For this review, take the finished solid that the model builds, in its own axes (mm). Round coordinates to 2 decimals unless told otherwise and drop trailing zeros. Loops run counter-clockwise (first coordinate to the right, second up) from the corner with the lowest first, then second, coordinate; pieces in that order, holes last. Notation, with made-up numbers: M -33,-22 L 1,-22 A20 ccw 1,6 Z; hole C -30,20.5 d9. An arc over 180 degrees is marked long. One line per question, with ' | ' between items. Start each with the question number.
1) We need section D-D (z = 15.5). Give the boundary of the cut face in (x, y), and give its area (3 significant figures).
2) For probe 1 along Z at (x, y) = (37.5, -1.25); probe 2 along X at (y, z) = (-0.25, 65); probe 3 along X at (y, z) = (-4, 45.5), list the stretches that pass through material, from the lowest coordinate up. Write a range as from..to.
3) For pin 1 Ø5 at (x, y) = (11, 2) entering from +Z; pin 2 Ø1 at (x, z) = (30, 11.5) entering from +Y; pin 3 Ø8 at (y, z) = (-3.5, 21.5) entering from +X, all flat-tipped, find the tip position at first contact; note any pin that passes through.
4) We need section B-B (y = 0). Give the boundary of the cut face in (x, z).
5) We need section A-A (x = 30). Give the boundary of the cut face in (y, z).
6) Mouldability with a two-part tool opening along X and no side actions: class faces 1 (the face through (0.57, 6.9, -0.08)), 2 (the face through (59.43, 0.08, -6.9)), 3 (the face through (25, 0, 40)), 4 (the face through (23, 0, 7.5)) as pulls with the +X half, pulls with the -X half, needs draft (parallel to the pull), parting line crosses it, or undercut.
7) We need section C-C (x = 48). Give the boundary of the cut face in (y, z).
```python
from build123d import *

# Parameters (mm, degrees)
SKETCH1_W           = 15
SKETCH1_H           = 15
BOSS_EXTRUDE1_DEPTH = 60
SKETCH3_R           = 5
BOSS_EXTRUDE2_DEPTH = 66
FILLET1_R           = 2


with BuildPart() as part:
    # Sketch1 → Boss-Extrude1 (new body)
    with BuildSketch(Plane(origin=(0, 0, 0), x_dir=(0, 0, -1), z_dir=(1, 0, 0))):
        Rectangle(SKETCH1_W, SKETCH1_H)
    extrude(amount=BOSS_EXTRUDE1_DEPTH)

    # Sketch3 → Boss-Extrude2 (add)
    with BuildSketch(Plane.XY.offset(7.5)):
        with Locations((30, 0)):
            Circle(SKETCH3_R)
    extrude(amount=BOSS_EXTRUDE2_DEPTH)

    # Fillet1
    fillet1_edges = [part.edges().sort_by_distance(p)[0] for p in [
        (60, 0, -7.5),
        (60, -7.5, 0),
        (60, 0, 7.5),
        (0, -7.5, 0),
        (0, 0, -7.5),
        (0, 7.5, 0),
        (0, 0, 7.5),
        (60, 7.5, 0),
        (30, -7.5, 7.5),
        (30, -7.5, -7.5),
        (30, 7.5, -7.5),
        (30, 7.5, 7.5),
    ]]
    fillet(fillet1_edges, radius=FILLET1_R)


solid = part.part
```
Answers below:
1) outline: C 30,0 d10 | area: 78.5 mm^2
2) probe 1: -7.5..7.5 | probe 2: 25.01..34.99 | probe 3: 27..33
3) pin 1: z = 7.5 | pin 2: y = 5 | pin 3: x = 35
4) outline: M 0,-5.5 A2 ccw 2,-7.5 L 58,-7.5 A2 ccw 60,-5.5 L 60,5.5 A2 ccw 58,7.5 L 35,7.5 L 35,73.5 L 25,73.5 L 25,7.5 L 2,7.5 A2 ccw 0,5.5 Z
5) outline: M -7.5,-5.5 A2 ccw -5.5,-7.5 L 5.5,-7.5 A2 ccw 7.5,-5.5 L 7.5,5.5 A2 ccw 5.5,7.5 L 5,7.5 L 5,73.5 L -5,73.5 L -5,7.5 L -5.5,7.5 A2 ccw -7.5,5.5 Z
6) face 1: pulls with the -X half | face 2: pulls with the +X half | face 3: parting line crosses it | face 4: needs draft
7) outline: M -7.5,-5.5 A2 ccw -5.5,-7.5 L 5.5,-7.5 A2 ccw 7.5,-5.5 L 7.5,5.5 A2 ccw 5.5,7.5 L -5.5,7.5 A2 ccw -7.5,5.5 Z
